Autodesk Inventor part; units mm, degrees
ref_plane "YZ Plane" through (0, 0, 0) normal (1, 0, 0) x (0, 1, 0)
ref_plane "XZ Plane" through (0, 0, 0) normal (0, 1, 0) x (-1, 0, 0)
ref_plane "XY Plane" through (0, 0, 0) normal (0, 0, 1) x (1, 0, 0)
sketch "Sketch1" plane through (0, 0, 0) normal (0, 0, 1) x (1, 0, 0)
  line L0 (0, 0) -> (355.6, 0)
  line L1 (355.6, 0) -> (355.6, 25.4)
  line L2 (355.6, 25.4) -> (0, 25.4)
  line L3 (0, 25.4) -> (0, 0)
  dimension "d0" = 355.6
  dimension "d1" = 25.4
extrude "Extrusion1" add sketch "Sketch1" along normal blind 25.4
sketch "Sketch2" plane through (355.6, 0, 0) normal (1, 0, 0) x (0, 0, -1)
  line L0 (-22.225, 3.175) -> (-3.175, 3.175)
  line L1 (-3.175, 3.175) -> (-3.175, 22.225)
  line L2 (-3.175, 22.225) -> (-22.225, 22.225)
  line L3 (-22.225, 22.225) -> (-22.225, 3.175)
  line L4 (-22.225, 3.175) -> (-3.175, 22.225) construction
  line L5 (-3.175, 3.175) -> (-22.225, 22.225) construction
  point P0 (-12.7, 12.7)
  dimension "d4" = 19.05
  dimension "d5" = 19.05
extrude "Extrusion2" cut sketch "Sketch2" against normal blind 355.6
properties part number "west coast backfront"
Model file for the job. Use its own axes, mm. A direction names the side the tool comes from. Coordinates: 2 decimals unless noted, no trailing zeros. Loops run counter-clockwise (first coordinate to the right, second up) from the corner with the lowest first, then second, coordinate; pieces in that order, holes last. Notation, with made-up numbers: M 77,-23.5 L 123,-23.5 A16 cw 123,-5.5 Z; hole C -38.75,77.5 d7. An arc over 180 degrees is marked long. Use CSV: the item, a comma, the result in double quotes. Start each with the question number.
1. Band-saw the part on A-A, the plane y = 13.75. List the corners of the cut face in (x, z) (3 decimals).
2. Tool access for faces 1 (the flat face through (0, 2, 13)), 2 (the flat face through (180, 22.225, 13)): list every direction of +Z, -Z, +X, -X, +Y, -Y with a clear straight run to the whole face (end or side of a thin tool).
3. Two-plate mould, pull along Y, no slides. Class faces 3 (the flat face through (175, 13, 0)), 4 (the flat face through (180, 25.4, 13)), 5 (the flat face through (180, 13, 22.225)): pulls with the +Y half, pulls with the -Y half, needs draft (parallel to the pull), parting line crosses it, or undercut.
4. Probe probe 1 along Z at (x, y) = (295, 13) (3 decimals). List the from-to ranges inside material, lowest first. Write a range as [from, to].
5. Band-saw the part on C-C, the plane x = 205.5. List the corners of the cut face in (y, z) (3 decimals), then the cut area to 3 significant figures.
Entries:
1,outline,"M 0,0 L 355.6,0 L 355.6,3.175 L 0,3.175 Z; M 0,22.225 L 355.6,22.225 L 355.6,25.4 L 0,25.4 Z"
2,face 1,"+Z, -Z, -X, +Y, -Y"
2,face 2,"+X, -X"
3,face 3,"needs draft"
3,face 4,"pulls with the +Y half"
3,face 5,"undercut"
4,probe 1,"z = [0, 3.175], [22.225, 25.4]"
5,outline,"M 0,0 L 25.4,0 L 25.4,25.4 L 0,25.4 Z; hole M 3.175,3.175 L 22.225,3.175 L 22.225,22.225 L 3.175,22.225 Z"
5,area,"282 mm2"
